Read the model definition and answer for the solid it produces. Units are mm, in the model's axes. Face numbers are marked on the shaded views. Give positions to 0.01 mm unless a question says otherwise; leave off trailing zeros. Order: outer loops, then holes, each group sorted by start corner. A loop starts at its lowest first (then second) coordinate and runs counter-clockwise, first axis right, second up. Notation, with made-up numbers: (50.25, 20.25) - (99.25, 20.25) arc R22 cw to (99.25, 26.25) - close; hole circle Ø10 at (30.25, 5). An arc over 180 degrees is marked (long way). Write item = value, one per line.
```python
from build123d import *

# Parameters (mm, degrees)
SKETCH1_R                    = 21
SKETCH1_R_2                  = 16
SKETCH1_R_3                  = 11
BOSS_EXTRUDE1_DEPTH          = 4
SKETCH2_R                    = 2.05
CUT_EXTRUDE1_DEPTH           = 30.966648128
CHAMFER1_SIZE                = 0.2
CIRPATTERN1_COUNT            = 8
CHAMFER1_OF_CIRPATTERN1_SIZE = 0.2


with BuildPart() as part:
    # Sketch1 → Boss-Extrude1 (new body)
    # profile 1 of 2: a face of its own
    with BuildSketch(Plane(origin=(0, 0, 0), x_dir=(1, 0, 0), z_dir=(0, 1, 0))):
        with Locations(Location((0, 0, 0), (0, 0, 270))):
            Circle(SKETCH1_R)
        Circle(SKETCH1_R_2, mode=Mode.SUBTRACT)
    # profile 2 of 2: a face of its own
    with BuildSketch(Plane(origin=(0, 0, 0), x_dir=(1, 0, 0), z_dir=(0, 1, 0))):
        Circle(SKETCH1_R_2)
        with Locations(Location((0, 0, 0), (0, 0, 270))):
            Circle(SKETCH1_R_3, mode=Mode.SUBTRACT)
    extrude(amount=BOSS_EXTRUDE1_DEPTH)

    # Sketch2 → Cut-Extrude1 (cut, through all)
    with BuildSketch(Plane(origin=(0, 4, 0), x_dir=(1, 0, 0), z_dir=(0, 1, 0))):
        with Locations(Location((16, 0, 0), (0, 0, 270))):
            Circle(SKETCH2_R)
    cut_extrude1 = extrude(amount=-CUT_EXTRUDE1_DEPTH, mode=Mode.SUBTRACT)

    # Chamfer1
    chamfer1_edges = [part.edges().sort_by_distance(p)[0] for p in [
        (16, 0, -2.05),
        (16, 4, -2.05),
    ]]
    chamfer(chamfer1_edges, length=CHAMFER1_SIZE)

    # CirPattern1: Cut-Extrude1 ×8 about axis
    cirpattern1_axis = Axis((0, 0, 0), (0, 1, 0))
    for i in range(1, CIRPATTERN1_COUNT):
        add(cut_extrude1.rotate(cirpattern1_axis, i * 360 / CIRPATTERN1_COUNT), mode=Mode.SUBTRACT)

    # Chamfer1 of CirPattern1
    chamfer1_of_cirpattern1_edges = [part.edges().sort_by_distance(p)[0] for p in [
        (9.864139598, 0, -12.7632774),
        (9.864139598, 4, -12.7632774),
        (-2.05, 0, -16),
        (-2.05, 4, -16),
        (-12.7632774, 0, -9.864139598),
        (-12.7632774, 4, -9.864139598),
        (-16, 0, 2.05),
        (-16, 4, 2.05),
        (-9.864139598, 0, 12.7632774),
        (-9.864139598, 4, 12.7632774),
        (2.05, 0, 16),
        (2.05, 4, 16),
        (12.7632774, 0, 9.864139598),
        (12.7632774, 4, 9.864139598),
    ]]
    chamfer(chamfer1_of_cirpattern1_edges, length=CHAMFER1_OF_CIRPATTERN1_SIZE)


solid = part.part
```
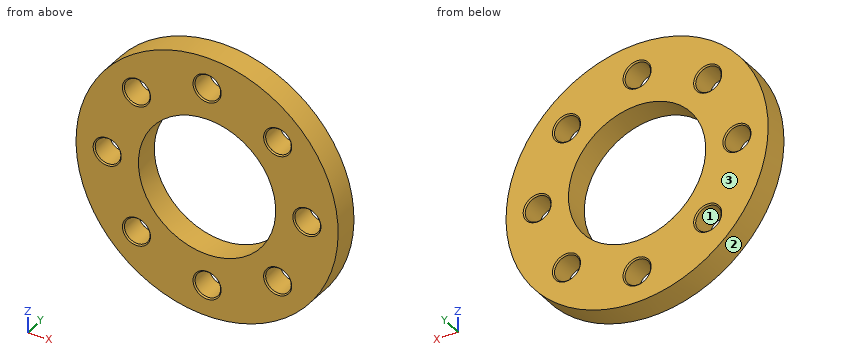
1. Section C-C (z = 16) is taken. Determine the outline of the cut face in (x, y).
Recorded:
outline = (-13.6, 0) - (-2.25, 0) - (-2.05, 0.2) - (-2.05, 3.8) - (-2.25, 4) - (-13.6, 4) - close; (2.05, 0.2) - (2.25, 0) - (13.6, 0) - (13.6, 4) - (2.25, 4) - (2.05, 3.8) - close
2. Section B-B (x = 4) is taken. Determine the outline of the cut face in (y, z).
Recorded:
outline = (0, -20.62) - (4, -20.62) - (4, -10.25) - (0, -10.25) - close; (0, 10.25) - (4, 10.25) - (4, 20.62) - (0, 20.62) - close
3. Flat-ended cylindrical pins translate along their axes: pin 1 (3.5 mm diameter, centred on x = 11.31, z = 11.31, fed in from -Y); pin 2 (1 mm diameter, centred on y = 1.5, z = 9.5, fed in from -X); pin 3 (5.5 mm diameter, centred on x = -11.31, z = 11.31, fed in from -Y); pin 4 (1 mm diameter, centred on x = -15, y = 0.5, fed in from -Z). Find the tip coordinate at first contact, or state that the pin passes through.
Recorded:
pin_1 = through
pin_2 = -18.97
pin_3 = 0
pin_4 = -15.19
4. Straight lines are drawn through the part: L1, parallel to X at y = 1.5, z = 0; L2, parallel to Z at x = -17, y = 2.4; L3, parallel to Z at x = -13, y = 3. For each, find the intervals that lie inside material, in ascending order. Write a range as [from, to].
Recorded:
L1 = [-21, -18.05], [-13.95, -11], [11, 13.95], [18.05, 21]
L2 = [-12.33, -1.79], [1.79, 12.33]
L3 = [-16.49, -12.48], [-10.15, 10.15], [12.48, 16.49]
5. Determine the mould class of the marked faces 1, 2 and 3 for opening direction X: +X half, -X half, draft (parallel to the pull), parting line (faces both ways), or undercut.
Recorded:
face_1 = undercut
face_2 = parting line
face_3 = draft
6. Section D-D (y = 2.45) is taken. Count the separate pieces of the cut face and the enclosed holes in it, and give its area (3 significant figures).
Recorded:
separate_pieces = 1
enclosed_holes = 9
area = 900 mm^2
7. Section A-A (z = 0) is taken. Determine the outline of the cut face in (x, y).
Recorded:
outline = (-21, 0) - (-18.25, 0) - (-18.05, 0.2) - (-18.05, 3.8) - (-18.25, 4) - (-21, 4) - close; (-13.95, 0.2) - (-13.75, 0) - (-11, 0) - (-11, 4) - (-13.75, 4) - (-13.95, 3.8) - close; (11, 0) - (13.75, 0) - (13.95, 0.2) - (13.95, 3.8) - (13.75, 4) - (11, 4) - close; (18.05, 0.2) - (18.25, 0) - (21, 0) - (21, 4) - (18.25, 4) - (18.05, 3.8) - close
